The listing builds one solid part. Answer for the finished solid, in the listing's coordinates (mm). Round coordinates to 2 decimals unless told otherwise and drop trailing zeros. Write each loop counter-clockwise with the first axis right and the second up, starting at its lowest first coordinate (ties: lowest second). Pieces come first, ordered by that corner, then holes.
Item 1: Find section B-B on y = -44.5. Give the vertices of the cut face in (x, z), then the cut area to 3 significant figures.
Item 2: Find section A-A on x = -2.5. Give the vertices of the cut face in (y, z).
Item 3: Find section C-C on z = 1.8. Give the vertices of the cut face in (x, y).
Item 4: Find the intervals of material crossed by probe 1 along Y at (x, z) = (-11, 2.35); probe 2 along Y at (x, z) = (25, 0.45); probe 3 along Y at (x, z) = (25.5, 1.5), in increasing order.
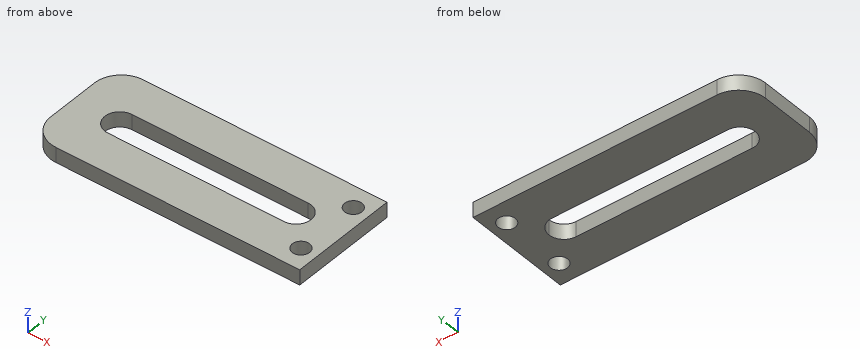
```python
from build123d import *

# Parameters (mm, degrees)
F0_W     = 50
F0_H     = 20
F0_R     = 1.6
F1_DEPTH = 2.8
F2_R     = 5


with BuildPart() as f1:
    # F0 (on Top) → F1 (new body)
    with BuildSketch(Plane.XY):
        with Locations((3.811439, -38.038712)):
            Rectangle(F0_W, F0_H)
        with Locations((25.811439, -44.038712)):
            Circle(F0_R, mode=Mode.SUBTRACT)
        with BuildLine():
            ThreePointArc((-12.459394, -40.788712), (-15.209394, -38.038712), (-12.459394, -35.288712))
            Line((-12.459394, -35.288712), (20.082271, -35.288712))
            ThreePointArc((20.082271, -35.288712), (22.026815, -36.094168), (22.832271, -38.038712))
            ThreePointArc((22.832271, -38.038712), (22.026815, -39.983256), (20.082271, -40.788712))
            Line((20.082271, -40.788712), (-12.459394, -40.788712))
        make_face(mode=Mode.SUBTRACT)
        with Locations((25.811439, -32.038712)):
            Circle(F0_R, mode=Mode.SUBTRACT)
    extrude(amount=F1_DEPTH)

    # F2
    f2_edges = [f1.edges().sort_by_distance(p)[0] for p in [
        (-21.188561, -48.038712, 1.4),
        (-21.188561, -28.038712, 1.4),
    ]]
    fillet(f2_edges, radius=F2_R)


solid = f1.part
```
Check values:
1. outline: (-20.97, 0) - (24.28, 0) - (24.28, 2.8) - (-20.97, 2.8) - close; (27.34, 0) - (28.81, 0) - (28.81, 2.8) - (27.34, 2.8) - close
1. area: 131 mm2
2. outline: (-48.04, 0) - (-40.79, 0) - (-40.79, 2.8) - (-48.04, 2.8) - close; (-35.29, 0) - (-28.04, 0) - (-28.04, 2.8) - (-35.29, 2.8) - close
3. outline: (-21.19, -43.04) arc R5 ccw to (-16.19, -48.04) - (28.81, -48.04) - (28.81, -28.04) - (-16.19, -28.04) arc R5 ccw to (-21.19, -33.04) - close; hole (-12.46, -40.79) - (20.08, -40.79) arc R2.75 ccw to (22.83, -38.04) arc R2.75 ccw to (20.08, -35.29) - (-12.46, -35.29) arc R2.75 ccw to start; hole circle Ø3.2 at (25.81, -44.04); hole circle Ø3.2 at (25.81, -32.04)
4. probe 1: y = -48.04 to -40.79, -35.29 to -28.04
4. probe 2: y = -48.04 to -45.42, -42.66 to -33.42, -30.66 to -28.04
4. probe 3: y = -48.04 to -45.61, -42.47 to -33.61, -30.47 to -28.04
